CAD build for the part. Positions are in the model's coordinates, mm. Face numbers are marked on the shaded views. Give positions to 0.01 mm unless a question says otherwise; leave off trailing zeros. Loops run counter-clockwise (first coordinate to the right, second up) from the corner with the lowest first, then second, coordinate; pieces in that order, holes last. Notation, with made-up numbers: M -21,-39.75 L 3,-39.75 A28 ccw 3,-3.75 Z; hole C 31.25,3 d3. An arc over 180 degrees is marked long. Answer as CSV lines item,"result".
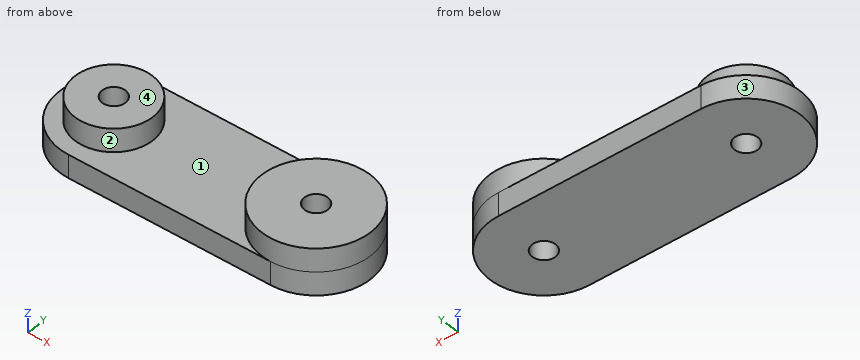
```python
from build123d import *

# Parameters (mm, degrees)
PAD_DEPTH         = 3
SKETCH001_R       = 7
SKETCH001_R_2     = 5
PAD001_DEPTH      = 3
SKETCH002_R       = 1.5
POCKET_DEPTH      = 3.001
POCKET_DEPTH_BACK = -3.001


with BuildPart() as part:
    # Sketch → Pad (new body)
    with BuildSketch(Plane.XY):
        with BuildLine():
            ThreePointArc((0, 7), (-7, 0), (0, -7))
            Line((0, -7), (26, -7))
            ThreePointArc((26, -7), (33, 0), (26, 7))
            Line((0, 7), (26, 7))
        make_face()
    extrude(amount=-PAD_DEPTH)

    # Sketch001 → Pad001 (join)
    with BuildSketch(Plane.XY):
        with Locations((26, 0)):
            Circle(SKETCH001_R)
        Circle(SKETCH001_R_2)
    extrude(amount=PAD001_DEPTH)

    # Sketch002 → Pocket (cut, two sides)
    with BuildSketch(Plane.XY) as pocket_sk:
        Circle(SKETCH002_R)
        with Locations((26, 0)):
            Circle(SKETCH002_R)
    extrude(amount=-POCKET_DEPTH, mode=Mode.SUBTRACT)
    extrude(pocket_sk.sketch, amount=-POCKET_DEPTH_BACK, mode=Mode.SUBTRACT)


solid = part.part
```
Q1. Cut at C-C (z = 2.35). Write the cut outline in (x, y).
Solution:
outline,"C 0,0 d10; C 26,0 d14; hole C 0,0 d3; hole C 26,0 d3"
Q2. Cut at D-D (x = 6). Write the cut outline in (y, z).
Solution:
outline,"M -7,-3 L 7,-3 L 7,0 L -7,0 Z"
Q3. Mould opens along X. For the marked faces 1, 2, 3 and 4 say: released by +X, released by -X, zero draft, split by the parting line, or undercut.
Solution:
face 1,"undercut"
face 2,"undercut"
face 3,"released by -X"
face 4,"zero draft"
Q4. Wall check: line 1 (Y direction, x = 26, z = 2.1); line 2 (X direction, y = -0.5, z = 0.3); line 3 (Z direction, x = 6.5, y = -1.25). Give the ranges that are in metal, low to high. Write a range as [from, to].
Solution:
line 1,"y = [-7, -1.5], [1.5, 7]"
line 2,"x = [-4.97, -1.41], [1.41, 4.97], [19.02, 24.59], [27.41, 32.98]"
line 3,"z = [-3, 0]"
Q5. Cut at A-A (y = 0). Write the cut outline in (x, z).
Solution:
outline,"M -7,-3 L -1.5,-3 L -1.5,3 L -5,3 L -5,0 L -7,0 Z; M 1.5,-3 L 24.5,-3 L 24.5,3 L 19,3 L 19,0 L 5,0 L 5,3 L 1.5,3 Z; M 27.5,-3 L 33,-3 L 33,3 L 27.5,3 Z"
Q6. Pin check, flat tip, straight feed: P1, Ø1, axis at y = -3.5, z = -0.5, coming from the -X side. Stop position of the tip, or through.
Solution:
P1,"stops at x = -6.32"
Q7. Cut at B-B (z = -0.75). Write the cut outline in (x, y), and give its area (3 significant figures).
Solution:
outline,"M 0,-7 L 26,-7 A7 ccw 26,7 L 0,7 A7 ccw Z; hole C 0,0 d3; hole C 26,0 d3"
area,"504 mm²"
